Here's how the part is built. I have some questions about the finished solid (model axes, mm). Round coordinates to 2 decimals unless told otherwise and drop trailing zeros. Write each loop counter-clockwise with the first axis right and the second up, starting at its lowest first coordinate (ties: lowest second). Pieces come first, ordered by that corner, then holes. Notation, with made-up numbers: (64.25, -9.5) - (80.25, -9.5) arc R19 ccw to (80.25, -3.5) - close; hole circle Ø2 at (-1.75, 8). An arc over 180 degrees is marked (long way). Return JSON: item names as keys, results as strings. Group by question number.
```python
from build123d import *

# Parameters (mm, degrees)
F1_DEPTH = 487.68
F3_DEPTH = 543.56
F4_R     = 25.4


# Not quite as in the source:
# - ends of sketch curves that miss each other by under 0.0002 mm in the source are joined


with BuildPart() as f1:
    # F0 (on Front) → F1 (new body, symmetric)
    with BuildSketch(Plane.XZ):
        Polygon((-83.2644920098, 41.3985210439), (60.6460442831, 41.3985210439), (60.6460442831, 104.8985210439), (-53.6539557169, 104.8985210439), align=None)
        Polygon((60.6460442831, 104.8985210439), (60.6460442831, 41.3985210439), (204.5565805759, 41.3985210439), (174.9460442831, 104.8985210439), align=None)
        Polygon((60.6460442831, 41.3985210439), (60.6460442831, -22.1014789561), (284.9671168688, -22.1014789561), (255.3565805759, 41.3985210439), (204.5565805759, 41.3985210439), align=None)
        Polygon((-163.6750283026, -22.1014789561), (60.6460442831, -22.1014789561), (60.6460442831, 41.3985210439), (-83.2644920098, 41.3985210439), (-134.0644920098, 41.3985210439), align=None)
        Polygon((-244.0855645955, -85.6014789561), (60.6460442831, -85.6014789561), (60.6460442831, -22.1014789561), (-163.6750283026, -22.1014789561), (-214.4750283026, -22.1014789561), align=None)
        Polygon((60.6460442831, -22.1014789561), (60.6460442831, -85.6014789561), (365.3776531616, -85.6014789561), (335.7671168688, -22.1014789561), (284.9671168688, -22.1014789561), align=None)
    extrude(amount=F1_DEPTH, both=True)

    # F2 (on Right) → F3 (cut, symmetric)
    with BuildSketch(Plane.YZ):
        Polygon((-396.5238630772, -85.6014788151), (-294.9238630772, -85.6014788151), (-265.3133267843, -22.1014788151), (-214.5133267843, -22.1014788151), (-184.9027904915, 41.3985211849), (-134.1027904915, 41.3985211849), (-104.4922541986, 104.8985211849), (-180.6922541986, 104.8985211849), (-487.68, 104.8985210439), (-487.68, -85.6014789561), align=None)
        Polygon((284.928818387, -22.1014788151), (314.5393546799, -85.6014788151), (487.68, -85.6014789561), (487.68, 104.8985210439), (124.1077458014, 104.8985210439), (153.7182820942, 41.3985211849), (204.5182820942, 41.3985211849), (234.128818387, -22.1014788151), align=None)
    extrude(amount=F3_DEPTH, both=True, mode=Mode.SUBTRACT)

    # F4
    f4_edges = [f1.edges().sort_by_distance(p)[0] for p in [
        (-68.459224, 138.913014, 73.148521),
        (-148.86976, 219.32355, 9.648521),
        (-229.280296, 299.734087, -53.851479),
        (350.572385, 299.734087, -53.851479),
        (270.161849, 219.32355, 9.648521),
        (189.751312, 138.913014, 73.148521),
        (350.572385, -280.118595, -53.851479),
        (270.161849, -199.708059, 9.648521),
        (189.751312, -119.297522, 73.148521),
        (-229.280296, -280.118595, -53.851479),
        (-148.86976, -199.708059, 9.648521),
        (-68.459224, -119.297522, 73.148521),
    ]]
    fillet(f4_edges, radius=F4_R)


solid = f1.part
```
1) Imagine slicing it at B-B (x = 3). Please give me the cut outline in (y, z), plus the area to 3 significant figures.
2) Imagine slicing it at C-C (y = -15). Please give me the cut outline in (x, z).
3) Imagine slicing it at D-D (y = -230). Please give me the cut outline in (x, z), plus the area to 3 significant figures.
4) Imagine slicing it at A-A (y = 161.5). Please give me the cut outline in (x, z), plus the area to 3 significant figures.
5) Will these pins go through, and if not, where does the flat tip stop? pin 1 Ø8 at (x, z) = (60, 58.5) entering from -Y; pin 2 Ø3 at (y, z) = (193.5, -6.5) entering from +X; pin 3 Ø15 at (x, y) = (-111, 5.5) entering from +Z.
6) If we mould it in two halves opening along Z, with no side actions, what happens to faces 1 (the cylindrical face through (-222.13, 292.234, -52.109)), 2 (the flat face through (56, 6, -85.601))? For each: released by +Z, released by -Z, zero draft, split by the parting line, or undercut.
7) I need wall thicknesses on line 1 along Z through (x, y) = (93.5, -227); line 2 along Z through (x, y) = (-13, -158); line 3 along Y through (x, z) = (-25.5, 82). Which ranges of each line are inside material? Lowest first, please.
Results found:
{
 "1": {"outline": "(-294.92, -85.6) - (314.54, -85.6) - (284.93, -22.1) - (234.13, -22.1) - (204.52, 41.4) - (153.72, 41.4) - (124.11, 104.9) - (-104.49, 104.9) - (-134.1, 41.4) - (-184.9, 41.4) - (-214.51, -22.1) - (-265.31, -22.1) - close", "area": "79,800 mm²"},
 "2": {"outline": "(-244.09, -85.6) - (365.38, -85.6) - (335.77, -22.1) - (284.97, -22.1) - (255.36, 41.4) - (204.56, 41.4) - (174.95, 104.9) - (-53.65, 104.9) - (-83.26, 41.4) - (-134.06, 41.4) - (-163.68, -22.1) - (-214.48, -22.1) - close"},
 "3": {"outline": "(-244.09, -85.6) - (365.38, -85.6) - (335.77, -22.1) - (-214.48, -22.1) - close", "area": "36,800 mm²"},
 "4": {"outline": "(-244.09, -85.6) - (365.38, -85.6) - (335.77, -22.1) - (284.97, -22.1) - (255.36, 41.4) - (-134.06, 41.4) - (-163.68, -22.1) - (-214.48, -22.1) - close", "area": "63,400 mm²"},
 "5": {"pin 1": "stops at y = -127.99", "pin 2": "stops at x = 278.39", "pin 3": "stops at z = 41.4"},
 "6": {"face 1": "released by +Z", "face 2": "released by -Z"},
 "7": {"line 1": "z = -85.6 to -22.1", "line 2": "z = -85.6 to 41.4", "line 3": "y = -115.17 to 134.79"}
}
